The drawing under review shows one solid part. Ordinate dimensions are in mm from its lowest x, y, z. A direction names the side the tool comes from. Give positions to 0.01 mm unless a question says otherwise; leave off trailing zeros. Write each loop counter-clockwise with the first axis right and the second up, starting at its lowest first coordinate (ties: lowest second). Pieces come first, ordered by that corner, then holes. Notation, with made-up numbers: (18, -32) - (37, -32) arc R22 ccw to (37, -15) - close; hole circle Ø4 at (-13, -14). An arc over 180 degrees is marked (long way). Write item = value, one per line.
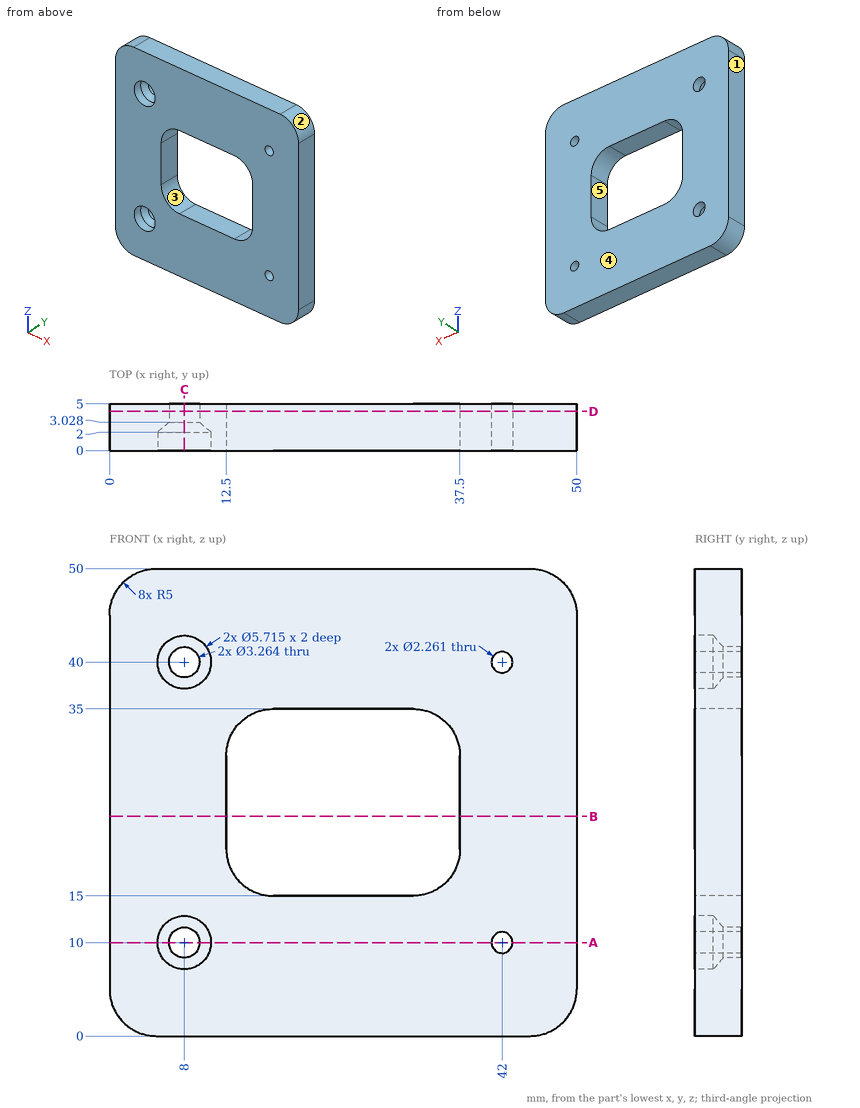
1. Draft analysis for pull direction X (two halves, no side actions). For the marked faces 1, 2 and 3, state which applies: +X half, -X half, draft (parallel to the pull), parting line (faces both ways), or undercut.
Findings below:
face_1 = -X half
face_2 = +X half
face_3 = undercut
2. Machinability: for the marked faces 4 and 5, which of the approach directions +Z, -Z, +X, -X, +Y, -Y give a long, thin tool a straight path to every point of the face, cutting with its end or side? Answer none if there is none.
Findings below:
face_4 = +Z, -Z, +X, -X, +Y
face_5 = +Y, -Y
3. Take a section at B-B on z = 23.5. Give the boundary of the cut face in (x, y).
Findings below:
outline = (0, 0) - (12.5, 0) - (12.5, 5) - (0, 5) - close; (37.5, 0) - (50, 0) - (50, 5) - (37.5, 5) - close
4. Insertion check: P1, Ø4, axis at x = 8, z = 40, coming from the -Y side; P2, Ø1.4, axis at x = 42, z = 10, coming from the +Y side. Each pin has a flat end and moves straight along its axis. Give the tip position at first contact, or say it passes through.
Findings below:
P1 = 2.72
P2 = through
5. Take a section at A-A on z = 10. Give the boundary of the cut face in (x, y).
Findings below:
outline = (0, 0) - (5.14, 0) - (5.14, 2) - (6.37, 3.03) - (6.37, 5) - (0, 5) - close; (9.63, 3.03) - (10.86, 2) - (10.86, 0) - (40.87, 0) - (40.87, 5) - (9.63, 5) - close; (43.13, 0) - (50, 0) - (50, 5) - (43.13, 5) - close
6. Take a section at C-C on x = 8. Give the boundary of the cut face in (y, z), and give its area (3 significant figures).
Findings below:
outline = (0, 0) - (5, 0) - (5, 8.37) - (3.03, 8.37) - (2, 7.14) - (0, 7.14) - close; (0, 12.86) - (2, 12.86) - (3.03, 11.63) - (5, 11.63) - (5, 38.37) - (3.03, 38.37) - (2, 37.14) - (0, 37.14) - close; (0, 42.86) - (2, 42.86) - (3.03, 41.63) - (5, 41.63) - (5, 50) - (0, 50) - close
area = 205 mm²
7. For line 1 (X direction, y = 4.65, z = 10); line 2 (Z direction, x = 42, y = 0.5); line 3 (Z direction, x = 8, y = 1.5), list the stretches that pass through material, from the lowest coordinate up. Write a range as from..to.
Findings below:
line_1 = 0..6.37, 9.63..40.87, 43.13..50
line_2 = 0..8.87, 11.13..38.87, 41.13..50
line_3 = 0..7.14, 12.86..37.14, 42.86..50
8. Take a section at D-D on y = 4.2. Give the boundary of the cut face in (x, z).
Findings below:
outline = (0, 5) arc R5 ccw to (5, 0) - (45, 0) arc R5 ccw to (50, 5) - (50, 45) arc R5 ccw to (45, 50) - (5, 50) arc R5 ccw to (0, 45) - close; hole circle Ø3.26 at (8, 10); hole circle Ø3.26 at (8, 40); hole (12.5, 20) arc R5 ccw to (17.5, 15) - (32.5, 15) arc R5 ccw to (37.5, 20) - (37.5, 30) arc R5 ccw to (32.5, 35) - (17.5, 35) arc R5 ccw to (12.5, 30) - close; hole circle Ø2.26 at (42, 10); hole circle Ø2.26 at (42, 40)
